Work out the finished part from the listing and answer in its coordinate system (mm). A direction names the side the tool comes from. Coordinates: 2 decimals unless noted, no trailing zeros. Write each loop counter-clockwise with the first axis right and the second up, starting at its lowest first coordinate (ties: lowest second). Pieces come first, ordered by that corner, then holes. Notation, with made-up numbers: (17, 66.25) - (30, 66.25) arc R21 cw to (30, 75.25) - close; hole circle Ø10 at (4, -6.75). An arc over 180 degrees is marked (long way). Use one line per item in the form item = value. Start each with the question number.
Item 1: Consider probe 1 along Y at (x, z) = (0, 9); probe 2 along Z at (x, y) = (-6.75, -0.25) (3 decimals). Determine where each line is inside the solid, lowest interval first.
Item 2: A cutting plane is placed at D-D (z = 12.5). Write down the section's boundary in (x, y) (1 decimal).
Item 3: Determine the mould class of faces 1 (the cylindrical face through (-1.72, -7.75, 12.53)), 2 (the flat face through (-4, -3, 15.875)), 3 (the cylindrical face through (3.78, -2.9, 7.83)) for opening direction X: released by +X, released by -X, zero draft, split by the parting line, or undercut.
Item 4: For faces 4 (the flat face through (-1, -5, 0)), 5 (the flat face through (7, 0, 9.525)), determine the directions among +Z, -Z, +X, -X, +Y, -Y from which every point of the face is accessible in a straight line to the end or side of a thin tool.
Item 5: Given pin 1 (1.5 mm diameter, centred on x = -1, z = 5.5, fed in from +Y); pin 2 (5 mm diameter, centred on x = -3.5, z = 13, fed in from -Y); pin 3 (5.5 mm diameter, centred on x = 0, y = 0, fed in from -Z); pin 4 (3 mm diameter, centred on y = -3.5, z = 11, fed in from -X), each flat-ended and moving along its own axis, determine where each tip first touches the part or whether it passes through.
Item 6: A cutting plane is placed at C-C (z = 4.5). Write down the section's boundary in (x, y) (1 decimal).
from build123d import *

# Parameters (mm, degrees)
SKETCH1_R                   = 7.9375
BOSS_EXTRUDE1_DEPTH         = 15.875
CHAMFER1_SIZE               = 0.254
SKETCH2_OUTSIDE_W           = 23.376
SKETCH2_OUTSIDE_H           = 23.376
SKETCH2_OUTSIDE_R           = 6.4643
CUT_EXTRUDE1_DEPTH          = 9.525
F_5_16_0_3125_DOWEL_HOLE1_D = 9.525


with BuildPart() as part:
    # Sketch1 → Boss-Extrude1 (new body)
    with BuildSketch(Plane.XY):
        Circle(SKETCH1_R)
    extrude(amount=BOSS_EXTRUDE1_DEPTH)

    # Chamfer1
    chamfer1_edges = [part.edges().sort_by_distance(p)[0] for p in [
        (-7.9375, 0, 15.875),
    ]]
    chamfer(chamfer1_edges, length=CHAMFER1_SIZE)

    # Sketch2 outside → Cut-Extrude1 (cut)
    with BuildSketch(Plane(origin=(0, 0, 0), x_dir=(-1, 0, 0), z_dir=(0, 0, -1))):
        Rectangle(SKETCH2_OUTSIDE_W, SKETCH2_OUTSIDE_H)
        Circle(SKETCH2_OUTSIDE_R, mode=Mode.SUBTRACT)
    extrude(amount=-CUT_EXTRUDE1_DEPTH, mode=Mode.SUBTRACT)

    # 5/16 (0.3125) Dowel Hole1 (through all)
    with Locations(Plane.XY.offset(15.875)):
        with Locations((0, 0)):
            Hole(F_5_16_0_3125_DOWEL_HOLE1_D / 2)


solid = part.part
Answer:
q1.probe_1 = -6.46 to -4.76, 4.76 to 6.46
q1.probe_2 = 9.525 to 15.875
q2.outline = circle Ø15.9 at (0, 0); hole circle Ø9.5 at (0, 0)
q3.face_1 = split by the parting line
q3.face_2 = zero draft
q3.face_3 = undercut
q4.face_4 = -Z, +X, -X, +Y, -Y
q4.face_5 = -Z
q5.pin_1 = 6.46
q5.pin_2 = -7.87
q5.pin_3 = through
q5.pin_4 = -7.68
q6.outline = circle Ø12.9 at (0, 0); hole circle Ø9.5 at (0, 0)
